For this review, take the finished solid that the model builds, in its own axes (mm). Face numbers are marked on the shaded views. A direction names the side the tool comes from. Give positions to 0.01 mm unless a question says otherwise; leave off trailing zeros. Loops run counter-clockwise (first coordinate to the right, second up) from the corner with the lowest first, then second, coordinate; pieces in that order, holes last. Notation, with made-up numbers: (-3, 41) - (22, 41) arc R22 cw to (22, 80) - close; hole circle Ø11 at (-8.75, -26.5). An arc over 180 degrees is marked (long way). Put each result on its own line as item: value.
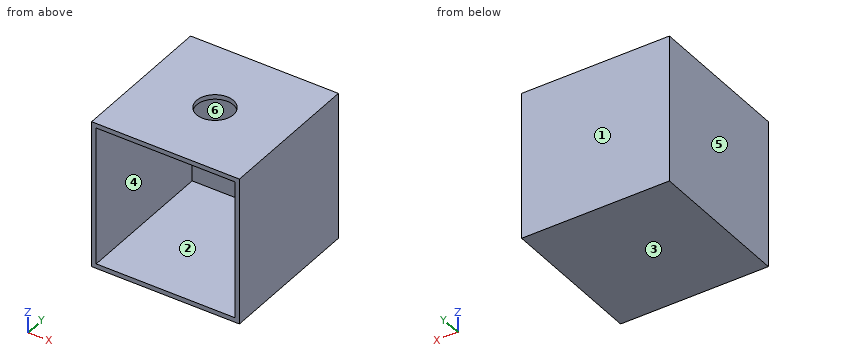
from build123d import *

# Parameters (mm, degrees)
F0_W     = 100
F0_H     = 100
F1_DEPTH = 100
F2_T     = -3.125
F3_R     = 12.5
F4_DEPTH = 3.125


with BuildPart() as f1:
    # F0 (on Top) → F1 (new body)
    with BuildSketch(Plane.XY):
        with Locations((-4.0166154504, 6.2387808433)):
            Rectangle(F0_W, F0_H)
    extrude(amount=F1_DEPTH)

    # F2
    f2_openings = [f1.faces().sort_by_distance(p)[0] for p in [
        (-4.016615, -43.761219, 50),
    ]]
    offset(amount=F2_T, openings=f2_openings)

    # F3 (on face) → F4 (cut, through all)
    with BuildSketch(Plane.XY.offset(100)):
        with Locations((-4.0166154504, 6.2387808433)):
            Circle(F3_R)
    extrude(amount=-F4_DEPTH, mode=Mode.SUBTRACT)


solid = f1.part
1) Draft analysis for pull direction Z (two halves, no side actions). For the marked faces 1, 2, 3 and 4, state which applies: pulls with the +Z half, pulls with the -Z half, needs draft (parallel to the pull), parting line crosses it, or undercut.
Geometry check:
face 1: needs draft
face 2: undercut
face 3: pulls with the -Z half
face 4: undercut
2) For the marked faces 5 and 6, list the 3-axis set-ups (+Z, -Z, +X, -X, +Y, -Y) from which the entire face can be reached by the end or side of a thin tool; tool diameter is ignored.
Geometry check:
face 5: +Z, -Z, -X, +Y, -Y
face 6: -Y
3) Take a section at C-C on z = 20.5. State the section outline as (x, y) points.
Geometry check:
outline: (-54.02, -43.76) - (-50.89, -43.76) - (-50.89, 53.11) - (42.86, 53.11) - (42.86, -43.76) - (45.98, -43.76) - (45.98, 56.24) - (-54.02, 56.24) - close
4) Insertion check: pin 1 Ø4 at (x, z) = (-6, 62.5) entering from -Y; pin 2 Ø15 at (x, y) = (-4.02, 6.24) entering from +Z (3 decimals). Each pin has a flat end and moves straight along its axis. Give the tip position at first contact, or say it passes through.
Geometry check:
pin 1: stops at y = 53.11
pin 2: stops at z = 3.125
5) Wall thickness on line 1 (X direction, y = -22, z = 13.5); line 2 (Z direction, x = -18, y = 46.5) (3 decimals); line 3 (Y direction, x = -36.5, z = 38.5): over which ranges is each line inside the solid? List them lowest first.
Geometry check:
line 1: x = -54.02 to -50.89, 42.86 to 45.98
line 2: z = 0 to 3.125, 96.875 to 100
line 3: y = 53.11 to 56.24
6) Take a section at D-D on y = -1. State the section outline as (x, z) points (3 decimals), and give its area (3 significant figures).
Geometry check:
outline: (-54.017, 0) - (45.983, 0) - (45.983, 100) - (6.174, 100) - (6.174, 96.875) - (42.858, 96.875) - (42.858, 3.125) - (-50.892, 3.125) - (-50.892, 96.875) - (-14.207, 96.875) - (-14.207, 100) - (-54.017, 100) - close
area: 1,150 mm²
7) Take a section at B-B on x = 39. State the section outline as (y, z) points (3 decimals), and give its area (3 significant figures).
Geometry check:
outline: (-43.761, 0) - (56.239, 0) - (56.239, 100) - (-43.761, 100) - (-43.761, 96.875) - (53.114, 96.875) - (53.114, 3.125) - (-43.761, 3.125) - close
area: 918 mm²
8) Take a section at A-A on y = 21. State the section outline as (x, z) points (3 decimals), and give its area (3 significant figures).
Geometry check:
outline: (-54.017, 0) - (45.983, 0) - (45.983, 100) - (-54.017, 100) - close; hole (-50.892, 3.125) - (42.858, 3.125) - (42.858, 96.875) - (-50.892, 96.875) - close
area: 1,210 mm²
